from build123d import *

# Parameters (mm, degrees)
EXTRUDE_1_DEPTH = 5


with BuildPart() as part:
    # ｽｹｯﾁ1 → ﾎﾞｽ - 押し出し1 (new body)
    with BuildSketch(Plane(origin=(0, 0, 0), x_dir=(0, 0, -1), z_dir=(1, 0, 0))):
        with BuildLine():
            Line((590.52, 8), (0, 8))
            ThreePointArc((0, 8), (-7.998416793, 0.159150236), (-0.31823748, -7.993667801))
            Line((-0.31823748, -7.993667801), (589.734351221, -31.484367383))
            ThreePointArc((589.734351221, -31.484367383), (610.266091459, -12.142902145), (590.52, 8))
        make_face()
        with BuildLine():
            ThreePointArc((-0.15911874, -3.9968339), (-3.999208397, 0.079575118), (0, 4))
            Line((0, 4), (590.52, 4))
            ThreePointArc((590.52, 4), (601.656931804, -0.613068196), (606.27, -11.75))
            ThreePointArc((606.27, -11.75), (601.43317213, -23.106283461), (589.893469961, -27.487533482))
            Line((589.893469961, -27.487533482), (-0.15911874, -3.9968339))
        make_face(mode=Mode.SUBTRACT)
    extrude(amount=EXTRUDE_1_DEPTH)


solid = part.part
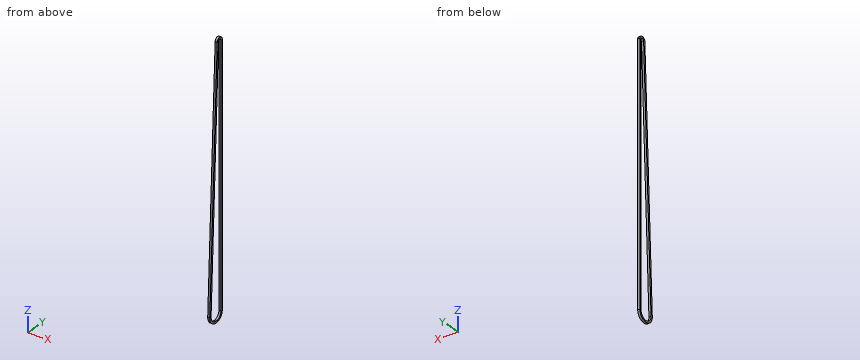
CAD build for the part. Positions are in the model's coordinates, mm. Round coordinates to 2 decimals unless told otherwise and drop trailing zeros. Loops run counter-clockwise (first coordinate to the right, second up) from the corner with the lowest first, then second, coordinate; pieces in that order, holes last. Notation, with made-up numbers: (-30.75, 85.25) - (-23.75, 85.25) arc R12 cw to (-23.75, 98.25) - close; hole circle Ø3 at (62, -13.75). An arc over 180 degrees is marked (long way). Put each result on its own line as item: value.
1. Slice it at A-A on z = -72. List the corners of the cut face in (x, y).
Geometry check:
outline: (0, -10.87) - (5, -10.87) - (5, -6.87) - (0, -6.87) - close; (0, 4) - (5, 4) - (5, 8) - (0, 8) - close
2. Wall check: line 1 (Y direction, x = 3.45, z = -166.5); line 2 (Y direction, x = 4.25, z = -52.5); line 3 (Z direction, x = 2.9, y = 0). Give the ranges that are in metal, low to high.
Geometry check:
line 1: -14.63 to -10.63, 4 to 8
line 2: -10.1 to -6.09, 4 to 8
line 3: -606.39 to -601.01, 4 to 8
3. Pin check, flat tips, straight feed: P1, Ø2.5, axis at x = 2.5, z = -435.5, coming from the -Y side; P2, Ø2, axis at x = 1.5, y = -17, coming from the -Z side. Stop position of each tip, or through.
Geometry check:
P1: y = -25.39
P2: z = -609.81
4. Slice it at B-B on x = 2.3. List the corners of the cut face in (y, z).
Geometry check:
outline: (-31.48, -589.73) arc R19.75 ccw (long way) to (8, -590.52) - (8, 0) arc R8 ccw to (-7.99, 0.32) - close; hole (-27.49, -589.89) arc R15.75 ccw (long way) to (4, -590.52) - (4, 0) arc R4 ccw to (-4, 0.16) - close
